Autodesk Inventor part; units mm, degrees
ref_plane "XZ Plane" through (0, 0, 0) normal (0, 1, 0) x (-1, 0, 0)
ref_plane "XY Plane" through (0, 0, 0) normal (0, 0, 1) x (1, 0, 0)
sketch "Skizze1" plane through (0, 0, 0) normal (0, 0, 1) x (1, 0, 0)
  circle A0 centre (0, 0) radius 10
  dimension "d0" = 20
extrude "Extrusion1" add sketch "Skizze1" along normal blind 5
sketch "Skizze2" plane through (0, 0, 5) normal (0, 0, 1) x (1, 0, 0)
  circle A0 centre (0, 0) radius 7.5
  circle A1 centre (0, 0) radius 10
  dimension "d3" = 15
extrude "Extrusion2" add sketch "Skizze2" along normal blind 14
sketch "Skizze3" plane through (0, 0, 0) normal (0, 0, -1) x (-1, 0, 0)
  circle A0 centre (0, 0) radius 2.45
  dimension "d6" = 4.9
extrude "Extrusion3" cut sketch "Skizze3" against normal blind 5
ref_plane "Arbeitsebene1" through (-10, 0, 0) normal (1, 0, 0) x (0, 1, 0)
sketch "Skizze7" plane through (0, 0, 19) normal (0, 0, 1) x (1, 0, 0)
  circle A0 centre (0, 0) radius 7.5
  circle A1 centre (0, 0) radius 10
extrude "Extrusion6" cut sketch "Skizze7" against normal blind 2
sketch "Skizze9" plane through (-10, 0, 0) normal (1, 0, 0) x (0, 1, 0)
  line L0 (-10, 17) -> (10, 17)
  line L1 (-0.2525, 8.5) -> (9.7475, 8.5)
  line L2 (-0.2525, 8.5) -> (-10.2525, 8.5)
  point P0 (0, 0)
  dimension "d36" = 8.5
hole "Bohrung3" at (-10, -0.2525, 8.5) direction (1, 0, 0) diameter 3.5 depth 8 tip angle 118
properties part number "2.2 Fuß"
For this review, take the finished solid that the model builds, in its own axes (mm). A direction names the side the tool comes from. Coordinates: 2 decimals unless noted, no trailing zeros. Order: outer loops, then holes, each group sorted by start corner. A loop starts at its lowest first (then second) coordinate and runs counter-clockwise, first axis right, second up. Notation, with made-up numbers: (63.5, 77.5) -> (70.5, 77.5) arc R25 ccw to (70.5, 104.5) -> close; hole circle Ø9 at (88, 54). An arc over 180 degrees is marked (long way). Return JSON: item names as keys, results as strings.
1. The part is to be moulded in two halves that separate along X. For faces 4 (the flat face through (-2, 2, 5)), 5 (the flat face through (2, -2, 0)), 6 (the cylindrical face through (9.54, -3, 8.38)), say which applies: +X half, -X half, draft (parallel to the pull), parting line (faces both ways), or undercut.
Answer block:
{"face 4": "undercut", "face 5": "draft", "face 6": "parting line"}
2. For line 1 (Y direction, x = 0, z = 1.6); line 2 (Y direction, x = 0, z = 11.5); line 3 (Z direction, x = -2.5, y = -1), list the stretches that pass through material, from the lowest coordinate up. Write a range as from..to.
Answer block:
{"line 1": "-10..-2.45, 2.45..10", "line 2": "-10..-7.5, 7.5..10", "line 3": "0..5"}
3. Machinability: for faces 1 (the cylindrical face through (-8.594, -1.435, 7.21)), 2 (the cylindrical face through (6.93, 2.87, 10.92)), 3 (the flat face through (4, 7, 17)), which of the approach directions +Z, -Z, +X, -X, +Y, -Y give a long, thin tool a straight path to every point of the face, cutting with its end or side? Answer none if there is none.
Answer block:
{"face 1": "-X", "face 2": "+Z", "face 3": "+Z, +X, -X, +Y, -Y"}
4. We need section D-D on x = -8.5. Write out the cut boundary in (y, z), and give its area (3 significant figures).
Answer block:
{"outline": "(-5.27, 0) -> (5.27, 0) -> (5.27, 17) -> (-5.27, 17) -> close; hole circle Ø3.5 at (-0.25, 8.5)", "area": "169 mm²"}
5. We need section A-A on x = 0. Write out the cut boundary in (y, z), and give its area (4 significant figures).
Answer block:
{"outline": "(-10, 0) -> (-2.45, 0) -> (-2.45, 5) -> (-7.5, 5) -> (-7.5, 17) -> (-10, 17) -> close; (2.45, 0) -> (10, 0) -> (10, 17) -> (7.5, 17) -> (7.5, 5) -> (2.45, 5) -> close", "area": "135.5 mm²"}
6. We need section C-C on z = 2. Write out the cut boundary in (x, y).
Answer block:
{"outline": "circle Ø20 at (0, 0); hole circle Ø4.9 at (0, 0)"}
7. We need section B-B on y = 1. Write out the cut boundary in (x, z), and give its area (3 significant figures).
Answer block:
{"outline": "(-9.95, 0) -> (-2.24, 0) -> (-2.24, 5) -> (-7.43, 5) -> (-7.43, 7.28) -> (-9.95, 7.28) -> close; (-9.95, 9.72) -> (-7.43, 9.72) -> (-7.43, 17) -> (-9.95, 17) -> close; (2.24, 0) -> (9.95, 0) -> (9.95, 17) -> (7.43, 17) -> (7.43, 5) -> (2.24, 5) -> close", "area": "131 mm²"}
8. For pin 1 Ø4 at (x, y) = (0, -0.5) entering from +Z; pin 2 Ø1.5 at (x, z) = (-6, 7.5) entering from +Y; pin 3 Ø1.5 at (x, z) = (1, 3.5) entering from +Y; pin 4 Ø4.5 at (x, y) = (0, 0) entering from -Z, all flat-tipped, find the tip position at first contact; note any pin that passes through.
Answer block:
{"pin 1": "z = 5", "pin 2": "y = 8.51", "pin 3": "y = 10", "pin 4": "through"}
